```python
from build123d import *

# Parameters (mm, degrees)
SKETCH1_W           = 100
SKETCH1_H           = 55
BOSS_EXTRUDE1_DEPTH = 5
SKETCH2_W           = 36
SKETCH2_H           = 53.5
SKETCH2_W_2         = 32
SKETCH2_H_2         = 49.5
SKETCH2_W_3         = 53.5
SKETCH2_H_3         = 36
SKETCH2_W_4         = 49.5
SKETCH2_H_4         = 32
EXTRUDE_THIN3_DEPTH = 5
SKETCH3_W           = 10
SKETCH3_H           = 14
CUT_EXTRUDE1_DEPTH  = 5
SKETCH4_W           = 14
SKETCH4_H           = 10
CUT_EXTRUDE2_DEPTH  = 5
SKETCH5_W           = 6
SKETCH5_H           = 28
SKETCH5_W_2         = 28
SKETCH5_H_2         = 6
CUT_EXTRUDE3_DEPTH  = 5
CUT_EXTRUDE4_DEPTH  = 10
SKETCH7_W           = 3.25
SKETCH7_H           = 5
CUT_EXTRUDE5_DEPTH  = 10


with BuildPart() as part:
    # Sketch1 → Boss-Extrude1 (new body)
    with BuildSketch(Plane.XY):
        Rectangle(SKETCH1_W, SKETCH1_H)
    extrude(amount=BOSS_EXTRUDE1_DEPTH)

    # Sketch2 → Extrude-Thin3 (add)
    # profile 1 of 2: a face of its own
    with BuildSketch(Plane.XY.offset(5)):
        with Locations((-25, 0)):
            Rectangle(SKETCH2_W, SKETCH2_H)
        with Locations((-25, 0)):
            Rectangle(SKETCH2_W_2, SKETCH2_H_2, mode=Mode.SUBTRACT)
    # profile 2 of 2: a face of its own
    with BuildSketch(Plane.XY.offset(5)):
        with Locations((20, 0)):
            Rectangle(SKETCH2_W_3, SKETCH2_H_3)
        with Locations((20, 0)):
            Rectangle(SKETCH2_W_4, SKETCH2_H_4, mode=Mode.SUBTRACT)
    extrude(amount=EXTRUDE_THIN3_DEPTH)

    # Sketch3 → Cut-Extrude1 (cut)
    with BuildSketch(Plane.XY.offset(5)):
        with BuildLine():
            ThreePointArc((-25, 24), (-32.071067812, 21.071067812), (-35, 14))
            Line((-35, 14), (-25, 14))
            Line((-25, 14), (-25, 24))
        make_face()
        with BuildLine():
            Line((-25, 24), (-25, 14))
            Line((-25, 14), (-15, 14))
            ThreePointArc((-15, 14), (-17.928932188, 21.071067812), (-25, 24))
        make_face()
        with Locations((-30, 7)):
            Rectangle(SKETCH3_W, SKETCH3_H)
        with Locations((-20, 7)):
            Rectangle(SKETCH3_W, SKETCH3_H)
        with Locations((-20, -7)):
            Rectangle(SKETCH3_W, SKETCH3_H)
        with Locations((-30, -7)):
            Rectangle(SKETCH3_W, SKETCH3_H)
        with BuildLine():
            Line((-25, -14), (-35, -14))
            ThreePointArc((-35, -14), (-32.071067812, -21.071067812), (-25, -24))
            Line((-25, -24), (-25, -14))
        make_face()
        with BuildLine():
            Line((-15, -14), (-25, -14))
            Line((-25, -14), (-25, -24))
            ThreePointArc((-25, -24), (-17.928932188, -21.071067812), (-15, -14))
        make_face()
    extrude(amount=-CUT_EXTRUDE1_DEPTH, mode=Mode.SUBTRACT)

    # Sketch4 → Cut-Extrude2 (cut)
    with BuildSketch(Plane.XY.offset(5)):
        with Locations((13, 5)):
            Rectangle(SKETCH4_W, SKETCH4_H)
        with Locations((27, 5)):
            Rectangle(SKETCH4_W, SKETCH4_H)
        with Locations((27, -5)):
            Rectangle(SKETCH4_W, SKETCH4_H)
        with Locations((13, -5)):
            Rectangle(SKETCH4_W, SKETCH4_H)
        with BuildLine():
            Line((6, 0), (6, 10))
            ThreePointArc((6, 10), (-1.071067812, 7.071067812), (-4, 0))
            Line((-4, 0), (6, 0))
        make_face()
        with BuildLine():
            Line((6, -10), (6, 0))
            Line((6, 0), (-4, 0))
            ThreePointArc((-4, 0), (-1.071067812, -7.071067812), (6, -10))
        make_face()
        with BuildLine():
            ThreePointArc((44, 0), (41.071067812, 7.071067812), (34, 10))
            Line((34, 10), (34, 0))
            Line((34, 0), (44, 0))
        make_face()
        with BuildLine():
            Line((44, 0), (34, 0))
            Line((34, 0), (34, -10))
            ThreePointArc((34, -10), (41.071067812, -7.071067812), (44, 0))
        make_face()
    extrude(amount=-CUT_EXTRUDE2_DEPTH, mode=Mode.SUBTRACT)

    # Sketch5 → Cut-Extrude3 (cut)
    with BuildSketch(Plane.XY.offset(5)):
        with Locations((-12, 0)):
            Rectangle(SKETCH5_W, SKETCH5_H)
        with Locations((-38, 0)):
            Rectangle(SKETCH5_W, SKETCH5_H)
        with Locations((20, 13)):
            Rectangle(SKETCH5_W_2, SKETCH5_H_2)
        with Locations((20, -13)):
            Rectangle(SKETCH5_W_2, SKETCH5_H_2)
    extrude(amount=-CUT_EXTRUDE3_DEPTH, mode=Mode.SUBTRACT)

    # Sketch6 → Cut-Extrude4 (cut)
    with BuildSketch(Plane.XY.offset(5)):
        Polygon((-50, 27.5), (-50, -27.5), (50, -27.5), (50, -18), (-6.75, -18), (-6.75, -15.188993876), (-7, -15.188993876), (-7, -26.75), (-43, -26.75), (-43, 26.75), (-7, 26.75), (-7, 18), (46.75, 18), (46.75, -15.188993876), (50, -15.188993876), (50, 27.5), align=None)
    extrude(amount=-CUT_EXTRUDE4_DEPTH, mode=Mode.SUBTRACT)

    # Sketch7 → Cut-Extrude5 (cut)
    with BuildSketch(Plane(origin=(0, -15.188993876, 0), x_dir=(1, 0, 0), z_dir=(0, 1, 0))):
        with Locations((48.375, -2.5)):
            Rectangle(SKETCH7_W, SKETCH7_H)
    extrude(amount=-CUT_EXTRUDE5_DEPTH, mode=Mode.SUBTRACT)


solid = part.part
```
The model under review builds one solid part; all positions refer to its coordinate system, in mm. A direction names the side the tool comes from. Give positions to 0.01 mm unless a question says otherwise; leave off trailing zeros. Write each loop counter-clockwise with the first axis right and the second up, starting at its lowest first coordinate (ties: lowest second). Pieces come first, ordered by that corner, then holes. Notation, with made-up numbers: (-9, 7) -> (17, 7) arc R22 ccw to (17, 34) -> close; hole circle Ø6 at (14.5, 64.25). An arc over 180 degrees is marked (long way). Put each result on its own line as item: value.
(1) We need section C-C, the plane x = 20. Give the boundary of the cut face in (y, z), and give its area (3 significant figures).
Results are:
outline: (-18, 0) -> (-16, 0) -> (-16, 10) -> (-18, 10) -> close; (16, 0) -> (18, 0) -> (18, 10) -> (16, 10) -> close
area: 40.0 mm²
(2) We need section A-A, the plane z = 8. Give the boundary of the cut face in (x, y).
Results are:
outline: (-43, -26.75) -> (-7, -26.75) -> (-7, 26.75) -> (-43, 26.75) -> close; (-6.75, -18) -> (46.75, -18) -> (46.75, 18) -> (-6.75, 18) -> close; hole (-41, -24.75) -> (-9, -24.75) -> (-9, 24.75) -> (-41, 24.75) -> close; hole (-4.75, -16) -> (44.75, -16) -> (44.75, 16) -> (-4.75, 16) -> close
(3) To check wall thickness, follow probe 1 along X at (y, z) = (-1.5, 8.75); probe 2 along Y at (x, z) = (-20, 7.5); probe 3 along Y at (x, z) = (8.5, 6.5). State the ranges of each line that lie inside material, in increasing order. Write a range as from..to.
Results are:
probe 1: -43..-41, -9..-7, -6.75..-4.75, 44.75..46.75
probe 2: -26.75..-24.75, 24.75..26.75
probe 3: -18..-16, 16..18
(4) We need section B-B, the plane y = -8. Give the boundary of the cut face in (x, z), and give its area (3 significant figures).
Results are:
outline: (-43, 0) -> (-41, 0) -> (-41, 10) -> (-43, 10) -> close; (-9, 0) -> (0, 0) -> (0, 5) -> (-4.75, 5) -> (-4.75, 10) -> (-6.75, 10) -> (-6.75, 5) -> (-7, 5) -> (-7, 10) -> (-9, 10) -> close; (40, 0) -> (46.75, 0) -> (46.75, 10) -> (44.75, 10) -> (44.75, 5) -> (40, 5) -> close
area: 129 mm²
(5) Tool access review of faces 5 (the flat face through (-41, 0, 6)), 6 (the flat face through (19, 18, 5)), 7 (the flat face through (6, 13, 3)): name each direction out of +Z, -Z, +X, -X, +Y, -Y from which nothing blocks a thin tool from reaching the whole face with its end or side.
Results are:
face 5: +Z
face 6: +Z, -Z, +X, +Y
face 7: +Z, -Z
(6) For pin 1 Ø3 at (x, z) = (25.5, 3) entering from -Y; pin 2 Ø3 at (x, z) = (14.5, 6.5) entering from +Y; pin 3 Ø5.5 at (x, y) = (41.5, -4.5) entering from +Z, all flat-tipped, find the tip position at first contact; note any pin that passes through.
Results are:
pin 1: y = -18
pin 2: y = 18
pin 3: z = 5
(7) We need section D-D, the plane y = -20. Give the boundary of the cut face in (x, z), and give its area (3 significant figures).
Results are:
outline: (-43, 0) -> (-33, 0) -> (-33, 5) -> (-41, 5) -> (-41, 10) -> (-43, 10) -> close; (-17, 0) -> (-7, 0) -> (-7, 10) -> (-9, 10) -> (-9, 5) -> (-17, 5) -> close
area: 120 mm²
(8) The part is to be moulded in two halves that separate along Y. For faces 1 (the flat face through (-25, 26.75, 5)), 2 (the flat face through (-6.75, 0, 7)), 3 (the flat face through (6, -13, 3)), 4 (the flat face through (-25, -24.75, 7)), say which applies: pulls with the +Y half, pulls with the -Y half, needs draft (parallel to the pull), parting line crosses it, or undercut.
Results are:
face 1: pulls with the +Y half
face 2: needs draft
face 3: undercut
face 4: undercut
